Check sheet for the modelled part. Datum: model origin and axes. Units: mm. Face numbers are marked on the shaded views. A direction names the side the tool comes from. Round coordinates to 2 decimals unless told otherwise and drop trailing zeros. Order: outer loops, then holes, each group sorted by start corner. A loop starts at its lowest first (then second) coordinate and runs counter-clockwise, first axis right, second up.
(1) Sectioned sample at A-A, the plane x = -17.5. Enter the section's corners in (y, z).
(2) Sectioned sample at D-D, the plane x = -8.5. Enter the section's corners in (y, z).
(3) Depth check by flat-ended pin: pin 1 (3.5 mm diameter, centred on x = -29, y = 8, fed in from -Z). Enter the tip coordinate at first touch or a pass-through.
(4) Mould release check, pull along Y, two halves, no side actions. Record for the marked faces 4, 5 and 6: released by +Y, released by -Y, zero draft, split by the parting line, or undercut.
(5) Sectioned sample at C-C, the plane x = -29. Enter the section's corners in (y, z), and give its area (3 significant figures).
(6) Tool access check on the marked faces 1, 2 and 3. Record the directions out of +Z, -Z, +X, -X, +Y, -Y that give a thin tool (end or side, any length) a straight path to the whole face; none if there is none.
(7) Thickness scan on probe 1 along X at (y, z) = (6, 2.05); probe 2 along Y at (x, z) = (-15.5, 3.5); probe 3 along Y at (x, z) = (-17.5, 0.55). Record the ranges inside material, lowest first.
(8) Sectioned sample at B-B, the plane z = 5.45. Enter the section's corners in (x, y), and give its area (3 significant figures).
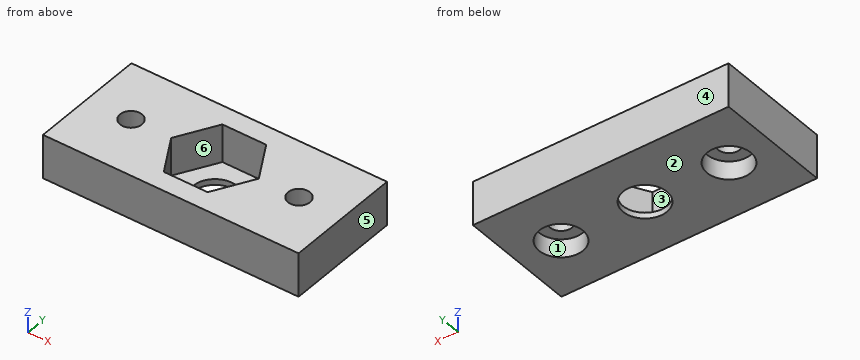
```python
from build123d import *

# Parameters (mm, degrees)
F0_W     = 35
F0_H     = 16
F0_R     = 1.5
F0_R_2   = 3
F1_DEPTH = 6
F3_DEPTH = 5.2
F4_R     = 3
F5_DEPTH = 2.5


with BuildPart() as f1:
    # F0 (on Top) → F1 (new body)
    with BuildSketch(Plane.XY):
        with Locations((-17.5, 8)):
            Rectangle(F0_W, F0_H)
        with Locations((-29, 8)):
            Circle(F0_R, mode=Mode.SUBTRACT)
        with Locations((-17.5, 8)):
            Circle(F0_R_2, mode=Mode.SUBTRACT)
        with Locations((-6, 8)):
            Circle(F0_R, mode=Mode.SUBTRACT)
    extrude(amount=F1_DEPTH)

    # F2 (on face) → F3 (cut)
    with BuildSketch(Plane.XY.offset(6)):
        with BuildLine():
            Line((-20.5, 2.7), (-17.5, 2.7))
            Line((-17.5, 2.7), (-17.5, 5))
            ThreePointArc((-17.5, 5), (-20.5, 8), (-17.5, 11))
            Line((-17.5, 11), (-17.5, 13.3))
            Line((-17.5, 13.3), (-20.5, 13.3))
            Line((-20.5, 13.3), (-23.5, 8))
            Line((-23.5, 8), (-20.5, 2.7))
        make_face()
        with BuildLine():
            ThreePointArc((-17.5, 11), (-15.37868, 10.12132), (-14.5, 8))
            Line((-14.5, 8), (-11.5, 8))
            Line((-11.5, 8), (-14.5, 13.3))
            Line((-14.5, 13.3), (-17.5, 13.3))
            Line((-17.5, 13.3), (-17.5, 11))
        make_face()
        with BuildLine():
            Line((-17.5, 5), (-17.5, 2.7))
            Line((-17.5, 2.7), (-14.5, 2.7))
            Line((-14.5, 2.7), (-11.5, 8))
            Line((-11.5, 8), (-14.5, 8))
            ThreePointArc((-14.5, 8), (-15.37868, 5.87868), (-17.5, 5))
        make_face()
    extrude(amount=-F3_DEPTH, mode=Mode.SUBTRACT)

    # F4 (on Top) → F5 (cut)
    with BuildSketch(Plane.XY):
        with Locations((-29, 8)):
            Circle(F4_R)
        with Locations((-6, 8)):
            Circle(F4_R)
    extrude(amount=F5_DEPTH, mode=Mode.SUBTRACT)


solid = f1.part
```
Derived:
1. outline: (0, 0) - (5, 0) - (5, 0.8) - (2.7, 0.8) - (2.7, 6) - (0, 6) - close; (11, 0) - (16, 0) - (16, 6) - (13.3, 6) - (13.3, 0.8) - (11, 0.8) - close
2. outline: (0, 0) - (6.34, 0) - (6.34, 2.5) - (9.66, 2.5) - (9.66, 0) - (16, 0) - (16, 6) - (0, 6) - close
3. pin 1: stops at z = 2.5
4. face 4: released by +Y
4. face 5: zero draft
4. face 6: undercut
5. outline: (0, 0) - (5, 0) - (5, 2.5) - (6.5, 2.5) - (6.5, 6) - (0, 6) - close; (9.5, 2.5) - (11, 2.5) - (11, 0) - (16, 0) - (16, 6) - (9.5, 6) - close
5. area: 70.5 mm2
6. face 1: -Z
6. face 2: -Z, +X, -X, +Y, -Y
6. face 3: +Z
7. probe 1: x = -35 to -31.24, -26.76 to -22.37, -12.63 to -8.24, -3.76 to 0
7. probe 2: y = 0 to 2.7, 13.3 to 16
7. probe 3: y = 0 to 5, 11 to 16
8. outline: (-35, 0) - (0, 0) - (0, 16) - (-35, 16) - close; hole circle Ø3 at (-29, 8); hole (-23.5, 8) - (-20.5, 2.7) - (-14.5, 2.7) - (-11.5, 8) - (-14.5, 13.3) - (-20.5, 13.3) - close; hole circle Ø3 at (-6, 8)
8. area: 450 mm2
